Could you check a few things on this model? Use its own coordinates, in mm. A direction names the side the tool comes from. Round coordinates to 2 decimals unless told otherwise and drop trailing zeros. Write each loop counter-clockwise with the first axis right and the second up, starting at its lowest first coordinate (ties: lowest second). Pieces come first, ordered by that corner, then holes. Notation, with made-up numbers: (89, -37) -> (108, -37) arc R36 ccw to (108, 0) -> close; hole circle Ø8 at (44, 44). An arc over 180 degrees is marked (long way). Return JSON: item names as keys, results as strings.
from build123d import *

# Parameters (mm, degrees)
F0_W      = 82.55
F0_H      = 38.1
F1_DEPTH  = 25.4
F2_W      = 57.15
F2_H      = 25.4
F3_DEPTH  = 25.4
F5_DEPTH  = 25.4
F7_DEPTH  = 25.4
F8_W      = 25.4
F8_H      = 25.4
F9_DEPTH  = 25.4
F10_R     = 12.7
F11_DEPTH = 25.4
F12_R     = 6.35
F13_DEPTH = 38.1
F14_DEPTH = 25.4


with BuildPart() as f1:
    # F0 (on Front) → F1 (new body)
    with BuildSketch(Plane.XZ):
        with Locations((5.1815754888, 19.05)):
            Rectangle(F0_W, F0_H)
    extrude(amount=-F1_DEPTH)

    # F2 (on Front) → F3 (cut)
    with BuildSketch(Plane.XZ):
        with Locations((17.8815754888, 25.4)):
            Rectangle(F2_W, F2_H)
    extrude(amount=-F3_DEPTH, mode=Mode.SUBTRACT)

    # F4 (on Top) → F5 (cut)
    with BuildSketch(Plane.XY):
        with BuildLine():
            ThreePointArc((33.7565754888, 25.4), (42.7368316099, 21.6802561211), (46.4565754888, 12.7))
            Line((46.4565754888, 12.7), (46.4565754888, 25.4))
            Line((46.4565754888, 25.4), (33.7565754888, 25.4))
        make_face()
        with BuildLine():
            ThreePointArc((46.4565754888, 12.7), (42.7368316099, 3.7197438789), (33.7565754888, 0))
            Line((33.7565754888, 0), (46.4565754888, 0))
            Line((46.4565754888, 0), (46.4565754888, 12.7))
        make_face()
    extrude(amount=F5_DEPTH, mode=Mode.SUBTRACT)

    # F6 (on Top) → F7 (cut)
    with BuildSketch(Plane.XY):
        with BuildLine():
            Line((28.8184100731, 19.05), (0, 19.05))
            ThreePointArc((0, 19.05), (-4.3434245112, 12.7), (0, 6.35))
            Line((0, 6.35), (29.70539537, 6.35))
            ThreePointArc((29.70539537, 6.35), (33.7396442751, 13.0127315686), (28.8184100731, 19.05))
        make_face()
    extrude(amount=F7_DEPTH, mode=Mode.SUBTRACT)

    # F8 (on face) → F9 (cut)
    with BuildSketch(Plane.XZ):
        with Locations((-23.3934245112, 25.4)):
            Rectangle(F8_W, F8_H)
    extrude(amount=-F9_DEPTH, mode=Mode.SUBTRACT)

    # F10 (on face) → F11 (join)
    with BuildSketch(Plane.XY.offset(12.7)):
        with Locations((-23.3934245112, 12.7)):
            Circle(F10_R)
    extrude(amount=F11_DEPTH)

    # F12 (on Top) → F13 (cut)
    with BuildSketch(Plane.XY):
        with Locations((-23.3934245112, 12.7)):
            Circle(F12_R)
    extrude(amount=F13_DEPTH, mode=Mode.SUBTRACT)

    # F14 (cut): faces of the model
    f14_faces = [f1.faces().sort_by_distance(p)[0] for p in [
        (-33.2566516865, 22.5632271754, 12.7),
        (-33.2566516865, 2.8367728246, 12.7),
    ]]
    extrude(f14_faces, amount=-F14_DEPTH, mode=Mode.SUBTRACT)


solid = f1.part
1) For faces 5 (the face through (-4.342, 12.814, 6.261)), 6 (the face through (-5, 13, 0)), which set-ups out of +Z, -Z, +X, -X, +Y, -Y let a thin tool reach every point of the face, with its end or its side?
Return value:
{"face 5": "+Z, -Z", "face 6": "-Z, +X, -X, +Y, -Y"}
2) Thinking about a two-plate mould opening in X: for faces 1 (the face through (-36.08, 13.26, 23.02)), 2 (the face through (15, 6.35, 6)), 3 (the face through (5, 0, 6)), 4 (the face through (15, 19.05, 6)), which applies, pulls with the +X half, pulls with the -X half, needs draft (parallel to the pull), parting line crosses it, or undercut?
Return value:
{"face 1": "parting line crosses it", "face 2": "undercut", "face 3": "needs draft", "face 4": "undercut"}
3) I want a section at C-C, the plane z = 33.5. Please give me the cut outline in (x, y), and give its area (3 significant figures).
Return value:
{"outline": "circle Ø25.4 at (-23.39, 12.7); hole circle Ø12.7 at (-23.39, 12.7)", "area": "380 mm²"}
4) I want a section at B-B, the plane y = 16.5. Please give me the cut outline in (x, z).
Return value:
{"outline": "(-35.51, 0) -> (-28.48, 0) -> (-28.48, 38.1) -> (-35.51, 38.1) -> close; (-18.31, 0) -> (-3.19, 0) -> (-3.19, 12.7) -> (-11.28, 12.7) -> (-11.28, 38.1) -> (-18.31, 38.1) -> close; (32.48, 0) -> (45.87, 0) -> (45.87, 12.7) -> (32.48, 12.7) -> close"}
5) I want a section at D-D, the plane y = 21. Please give me the cut outline in (x, z).
Return value:
{"outline": "(-33.01, 0) -> (43.37, 0) -> (43.37, 12.7) -> (-13.78, 12.7) -> (-13.78, 38.1) -> (-33.01, 38.1) -> close"}
6) I want a section at A-A, the plane x = 13. Please give me the cut outline in (y, z), and give its area (3 significant figures).
Return value:
{"outline": "(0, 0) -> (6.35, 0) -> (6.35, 12.7) -> (0, 12.7) -> close; (19.05, 0) -> (25.4, 0) -> (25.4, 12.7) -> (19.05, 12.7) -> close", "area": "161 mm²"}
7) Will these pins go through, and if not, where does the flat tip stop? pin 1 Ø3 at (x, y) = (-6.5, 10) entering from +Z; pin 2 Ø10 at (y, z) = (7, 17) entering from +X.
Return value:
{"pin 1": "z = 12.7", "pin 2": "x = 46.06"}
8) If I drill on probe 1 along Y at (x, z) = (-23, 20.5); probe 2 along X at (y, z) = (7.25, 9.5); probe 3 along Y at (x, z) = (9, 5), over which ranges is the centre line in solid material (lowest first)? Write a range as [from, to].
Return value:
{"probe 1": "[0.01, 6.36], [19.04, 25.39]", "probe 2": "[-34.86, -26.65], [-20.13, -1.62], [31.2, 45.23]", "probe 3": "[0, 6.35], [19.05, 25.4]"}
